from build123d import *

# Parameters (mm, degrees)
SKETCH1_W           = 60
SKETCH1_H           = 50
BOSS_EXTRUDE1_DEPTH = 4
SKETCH2_W           = 60
SKETCH2_H           = 4
BOSS_EXTRUDE2_DEPTH = 45
SKETCH3_W           = 40
SKETCH3_H           = 20
CUT_EXTRUDE1_DEPTH  = 60
SKETCH4_W           = 60
SKETCH4_H           = 31
CUT_EXTRUDE2_DEPTH  = 10
SKETCH5_R           = 2
CUT_EXTRUDE3_DEPTH  = 60.581876439
SKETCH6_R           = 1.81
CUT_EXTRUDE4_DEPTH  = 10
SKETCH7_R           = 1.81
CUT_EXTRUDE5_DEPTH  = 58.323642592


with BuildPart() as part:
    # Sketch1 → Boss-Extrude1 (new body)
    with BuildSketch(Plane.XY):
        Rectangle(SKETCH1_W, SKETCH1_H)
    extrude(amount=BOSS_EXTRUDE1_DEPTH)

    # Sketch2 → Boss-Extrude2 (add)
    with BuildSketch(Plane(origin=(0, 0, 0), x_dir=(-1, 0, 0), z_dir=(0, 0, -1))):
        with Locations((0, 23)):
            Rectangle(SKETCH2_W, SKETCH2_H)
    extrude(amount=BOSS_EXTRUDE2_DEPTH)

    # Sketch3 → Cut-Extrude1 (cut)
    with BuildSketch(Plane(origin=(0, 25, 0), x_dir=(1, 0, 0), z_dir=(0, 1, 0))):
        with Locations((0, 31)):
            Rectangle(SKETCH3_W, SKETCH3_H)
    extrude(amount=-CUT_EXTRUDE1_DEPTH, mode=Mode.SUBTRACT)

    # Sketch4 → Cut-Extrude2 (cut)
    with BuildSketch(Plane(origin=(0, 0, 0), x_dir=(-1, 0, 0), z_dir=(0, 0, -1))):
        with Locations((0, -9.5)):
            Rectangle(SKETCH4_W, SKETCH4_H)
    extrude(amount=-CUT_EXTRUDE2_DEPTH, mode=Mode.SUBTRACT)

    # Sketch5 → Cut-Extrude3 (cut, through all)
    with BuildSketch(Plane(origin=(0, 0, 0), x_dir=(-1, 0, 0), z_dir=(0, 0, -1))):
        with Locations((-15, 13.5)):
            Circle(SKETCH5_R)
        with Locations((15, 13.5)):
            Circle(SKETCH5_R)
    extrude(amount=-CUT_EXTRUDE3_DEPTH, mode=Mode.SUBTRACT)

    # Sketch6 → Cut-Extrude4 (cut)
    with BuildSketch(Plane(origin=(0, 25, 0), x_dir=(1, 0, 0), z_dir=(0, 1, 0))):
        with Locations(Location((23.9, 25, 0), (0, 0, 270))):
            Circle(SKETCH6_R)
        with Locations(Location((23.9, 37, 0), (0, 0, 270))):
            Circle(SKETCH6_R)
    extrude(amount=-CUT_EXTRUDE4_DEPTH, mode=Mode.SUBTRACT)

    # Sketch7 → Cut-Extrude5 (cut, through all)
    with BuildSketch(Plane(origin=(0, 25, 0), x_dir=(1, 0, 0), z_dir=(0, 1, 0))):
        with Locations(Location((-23.9, 37, 0), (0, 0, 270))):
            Circle(SKETCH7_R)
        with Locations(Location((-23.9, 25, 0), (0, 0, 270))):
            Circle(SKETCH7_R)
    extrude(amount=-CUT_EXTRUDE5_DEPTH, mode=Mode.SUBTRACT)


solid = part.part
Model file for the job. Use its own axes, mm. A direction names the side the tool comes from. Give positions to 0.01 mm unless a question says otherwise; leave off trailing zeros. Loops run counter-clockwise (first coordinate to the right, second up) from the corner with the lowest first, then second, coordinate; pieces in that order, holes last.
1) Flat gauge pins, fed straight in: pin 1 Ø1.5 at (x, y) = (-6, 12) entering from -Z; pin 2 Ø4.5 at (x, z) = (-23.9, -25) entering from -Y. Where does each tip first touch, or does it go through?
2) Pull direction Z, two halves, no side cores. Call faces 4 (the cylindrical face through (-23.82, 23.03, -38.81)), 5 (the flat face through (0, 14, 0)), 6 (the flat face through (0, 16, 4)), 7 (the flat face through (20, 23, -31)): +Z half, -Z half, draft (parallel to the pull), parting line (faces both ways), or undercut.
3) Saw through at A-A (z = -25). Write the cut outline in (x, y).
4) Wall check: line 1 (X direction, y = 21.85, z = -37); line 2 (Z direction, x = -18.5, y = 22.25); line 3 (Y direction, x = -24.5, z = -32.5). Give the ranges that are in metal, low to high.
5) Saw through at D-D (x = -23.9). Write the cut outline in (y, z), plus the area to 3 significant figures.
6) Saw through at B-B (y = 13.5). Write the cut outline in (x, z), plus the area to 3 significant figures.
7) Tool access for faces 1 (the flat face through (0, 23, -41)), 2 (the flat face through (30, 22, -17)), 3 (the flat face through (0, 21, -17)): list every direction of +Z, -Z, +X, -X, +Y, -Y with a clear straight run to the whole face (end or side of a thin tool).
8) Saw through at C-C (x = 10.5). Write the cut outline in (y, z), plus the area to 3 significant figures.
Answer block:
1. pin 1: stops at z = 0
1. pin 2: stops at y = 21
2. face 4: undercut
2. face 5: -Z half
2. face 6: +Z half
2. face 7: undercut
3. outline: (-30, 21) - (-25.71, 21) - (-25.71, 25) - (-30, 25) - close; (-22.09, 21) - (-20, 21) - (-20, 25) - (-22.09, 25) - close; (20, 21) - (22.09, 21) - (22.09, 25) - (20, 25) - close; (25.71, 21) - (30, 21) - (30, 25) - (25.71, 25) - close
4. line 1: x = -30 to -25.71, -22.09 to -20, 20 to 22.09, 25.71 to 30
4. line 2: z = -45 to -41, -21 to 4
4. line 3: y = 21 to 25
5. outline: (6, 0) - (21, 0) - (21, -23.19) - (25, -23.19) - (25, 4) - (6, 4) - close; (21, -45) - (25, -45) - (25, -38.81) - (21, -38.81) - close; (21, -35.19) - (25, -35.19) - (25, -26.81) - (21, -26.81) - close
5. area: 227 mm2
6. outline: (-30, 0) - (-17, 0) - (-17, 4) - (-30, 4) - close; (-13, 0) - (13, 0) - (13, 4) - (-13, 4) - close; (17, 0) - (30, 0) - (30, 4) - (17, 4) - close
6. area: 208 mm2
7. face 1: +Y, -Y
7. face 2: +Z, -Z, +X, +Y, -Y
7. face 3: -Z, +X, -X, -Y
8. outline: (6, 0) - (21, 0) - (21, -21) - (25, -21) - (25, 4) - (6, 4) - close; (21, -45) - (25, -45) - (25, -41) - (21, -41) - close
8. area: 176 mm2
